Build history of the part. All positions in model axes, mm. Give positions to 0.01 mm unless a question says otherwise; leave off trailing zeros. Write each loop counter-clockwise with the first axis right and the second up, starting at its lowest first coordinate (ties: lowest second). Pieces come first, ordered by that corner, then holes. Notation, with made-up numbers: (-0.5, 73) -> (4.5, 73) arc R19 ccw to (4.5, 81) -> close; hole circle Ø1 at (73.5, 32). An arc over 180 degrees is marked (long way). One line per question, with ' | ' between items. Start each with the question number.
(1) Band-saw the part on A-A, the plane y = 0. Give the cut face in (x, z) (3 decimals), and give its area (3 significant figures).
(2) Pin check, flat tips, straight feed: P1, Ø2, axis at y = -1.5, z = -11, coming from the +X side; P2, Ø6, axis at y = -2.5, z = -4.5, coming from the +X side; P3, Ø5, axis at y = 3.5, z = -7.5, coming from the -X side. Stop position of each tip, or through.
(3) Pull direction Y, two halves, no side cores. Call faces 1 (the cylindrical face through (-1.08, 4.88, -8.84)), 2 (the flat face through (2, -5, -2)), 3 (the cylindrical face through (1.74, 0.55, -8.15)): released by +Y, released by -Y, zero draft, split by the parting line, or undercut.
(4) Band-saw the part on C-C, the plane z = -3. Give the cut face in (x, y) (3 decimals), and give its area (3 significant figures).
(5) Drill centre lines: probe 1 along Y at (x, z) = (0, -9.5) (3 decimals); probe 2 along X at (y, z) = (0.25, -3.75); probe 3 along X at (y, z) = (1.5, -9). Where is each one in solid material? Low to high. Write a range as from..to.
from build123d import *

# Parameters (mm, degrees)
F0_R     = 6.25
F0_R_2   = 1.825
F1_DEPTH = 16
F2_SIZE  = 1
F3_R     = 6.25
F3_R_2   = 5
F4_DEPTH = 14
F5_SIZE  = 0.5


with BuildPart() as f1:
    # F0 (on Top) → F1 (new body)
    with BuildSketch(Plane.XY):
        Circle(F0_R)
        Circle(F0_R_2, mode=Mode.SUBTRACT)
    extrude(amount=-F1_DEPTH)

    # F2
    f2_edges = [f1.edges().sort_by_distance(p)[0] for p in [
        (-1.825, 0, 0),
    ]]
    chamfer(f2_edges, length=F2_SIZE)

    # F3 (on face) → F4 (cut)
    with BuildSketch(Plane(origin=(0, 0, -16), x_dir=(1, 0, 0), z_dir=(0, 0, -1))):
        Circle(F3_R)
        Circle(F3_R_2, mode=Mode.SUBTRACT)
    extrude(amount=-F4_DEPTH, mode=Mode.SUBTRACT)

    # F5
    f5_edges = [f1.edges().sort_by_distance(p)[0] for p in [
        (-5, 0, -16),
        (-1.825, 0, -16),
        (-6.25, 0, 0),
    ]]
    chamfer(f5_edges, length=F5_SIZE)


solid = f1.part
Results:
1) outline: (-6.25, -2) -> (-5, -2) -> (-5, -15.5) -> (-4.5, -16) -> (-2.325, -16) -> (-1.825, -15.5) -> (-1.825, -1) -> (-2.825, 0) -> (-5.75, 0) -> (-6.25, -0.5) -> close; (1.825, -15.5) -> (2.325, -16) -> (4.5, -16) -> (5, -15.5) -> (5, -2) -> (6.25, -2) -> (6.25, -0.5) -> (5.75, 0) -> (2.825, 0) -> (1.825, -1) -> close | area: 105 mm²
2) P1: stops at x = 4.97 | P2: stops at x = 6.19 | P3: stops at x = -4.9
3) face 1: split by the parting line | face 2: zero draft | face 3: undercut
4) outline: circle Ø10 at (0, 0); hole circle Ø3.65 at (0, 0) | area: 68.1 mm²
5) probe 1: y = -5..-1.825, 1.825..5 | probe 2: x = -4.99..-1.81, 1.81..4.99 | probe 3: x = -4.77..-1.04, 1.04..4.77
